```python
from build123d import *

# Parameters (mm, degrees)
ESQUISSE1_R             = 2.85
SHAPE_DEPTH             = 20.85
ESQUISSE2_R             = 4.35
BOSS_EXTRU_2_DEPTH      = 2
ESQUISSE3_R             = 3.2
ENL_V_MAT_EXTRU_1_DEPTH = 1
CONG_1_R                = 2
ESQUISSE4_R             = 0.8
ALIGNBEAM_DEPTH         = 0.8


with BuildPart() as part:
    # Esquisse1 → Shape (new body)
    with BuildSketch(Plane.XY):
        Circle(ESQUISSE1_R)
    extrude(amount=SHAPE_DEPTH)

    # Esquisse2 → Boss.-Extru.2 (add)
    with BuildSketch(Plane.XY.offset(20.85)):
        Circle(ESQUISSE2_R)
    extrude(amount=BOSS_EXTRU_2_DEPTH)

    # Esquisse3 → Enlèv. mat.-Extru.1 (cut)
    with BuildSketch(Plane.XY.offset(22.85)):
        Circle(ESQUISSE3_R)
    extrude(amount=-ENL_V_MAT_EXTRU_1_DEPTH, mode=Mode.SUBTRACT)

    # Congé1
    # the kernel refuses this fillet: 2 mm, written as the material it adds along each edge
    with BuildSketch(Plane(origin=(0, 0, 20.85), x_dir=(1, 0, 0), z_dir=(0, -1, 0))) as cong_1_piece_1:
        with BuildLine():
            CenterArc((4.85, -1.936491673), CONG_1_R, 104.477512186, 75.522487814)
            Line((2.85, -1.936491673), (2.81, -1.936491673))
            Line((2.81, -1.936491673), (2.81, 0))
            Line((2.81, 0), (2.85, 0.04))
            ThreePointArc((2.85, 0.04), (3.6, 0.04), (4.34, 0.038729833))
            Line((4.34, 0.038729833), (4.35, 0))
        make_face()
    revolve(axis=Axis((0, 0, 20.85), (0, 0, 1)))

    # Esquisse4 → AlignBeam (add)
    with BuildSketch(Plane(origin=(0, 0, 0), x_dir=(-1, 0, 0), z_dir=(0, 0, -1))):
        Circle(ESQUISSE4_R)
    extrude(amount=ALIGNBEAM_DEPTH)


solid = part.part
```
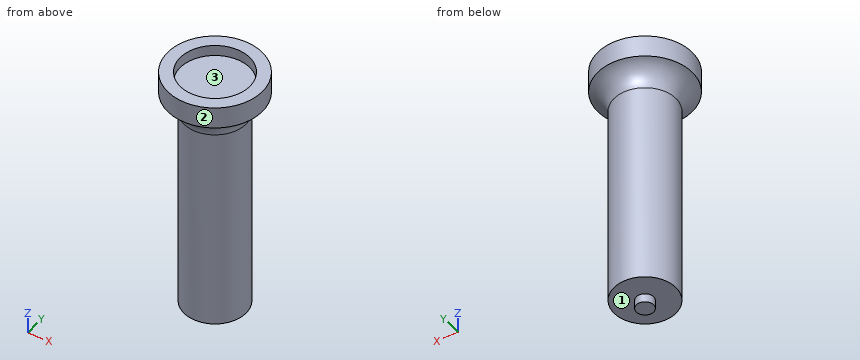
Source: CAD feature listing. Evaluate the final solid. Frame: model axes, mm. Face numbers are marked on the shaded views. Give positions to 0.01 mm unless a question says otherwise; leave off trailing zeros. Loops run counter-clockwise (first coordinate to the right, second up) from the corner with the lowest first, then second, coordinate; pieces in that order, holes last. Notation, with made-up numbers: (76.25, 72) - (102.25, 72) arc R11 cw to (102.25, 79) - close; hole circle Ø11 at (-33.5, -14.5). An arc over 180 degrees is marked (long way). Use CSV: the item, a comma, the result in double quotes. Start each with the question number.
1. Ray query, L1, parallel to Y at x = 0, z = 22.2; L2, parallel to Z at x = -0.5, y = 2; L3, parallel to Z at x = 1.5, y = -2.75. Return the intervals inside material, ascending.
2. Draft query along Y for the marked faces 1, 2 and 3. Return one class per face: +Y half, -Y half, draft (parallel to the pull), parting line (faces both ways), or undercut.
3. Section C-C (z = 10). Output: boundary loops of the cut face in (x, y).
4. Pin query (flat end, axial travel): pin 1 (1.9 mm diameter, centred on x = 0.5, y = 0, fed in from +Z); pin 2 (3 mm diameter, centred on x = 2, z = 15, fed in from -Y); pin 3 (5 mm diameter, centred on x = 2, z = 9.5, fed in from +Y). Return the tip coordinate at first contact, or that it passes through.
5. Section A-A (y = 0). Output: boundary loops of the cut face in (x, z).
Response:
1,L1,"-4.35 to -3.2, 3.2 to 4.35"
1,L2,"0 to 21.85"
1,L3,"19.94 to 21.85"
2,face 1,"draft"
2,face 2,"parting line"
2,face 3,"undercut"
3,outline,"circle Ø5.7 at (0, 0)"
4,pin 1,"z = 21.85"
4,pin 2,"y = -2.81"
4,pin 3,"y = 2.85"
5,outline,"(-4.35, 20.85) arc R2 cw to (-2.85, 18.91) - (-2.85, 0) - (-0.8, 0) - (-0.8, -0.8) - (0.8, -0.8) - (0.8, 0) - (2.85, 0) - (2.85, 18.91) arc R2 cw to (4.35, 20.85) - (4.35, 22.85) - (3.2, 22.85) - (3.2, 21.85) - (-3.2, 21.85) - (-3.2, 22.85) - (-4.35, 22.85) - close"
